Verification items for the finished model (mm, model axes). Face numbers are marked on the shaded views. A direction names the side the tool comes from. Coordinates: 2 decimals unless noted, no trailing zeros. Write each loop counter-clockwise with the first axis right and the second up, starting at its lowest first coordinate (ties: lowest second). Pieces come first, ordered by that corner, then holes. Notation, with made-up numbers: (37, 50.5) -> (56, 50.5) arc R33 cw to (56, 81.5) -> close; hole circle Ø10 at (15.5, 86.5). An arc over 180 degrees is marked (long way). Write item = value, one per line. Start each with the question number.
(1) Section check A-A (z = -26). Record the cut outline in (x, y), plus the area to 3 significant figures.
(2) Section check C-C (y = 25.5). Record the cut outline in (x, z).
(3) Gauge pin test, flat ends, axial feed: pin 1 Ø3 at (x, z) = (2.92, -26) entering from +Y; pin 2 Ø4 at (y, z) = (26.27, -13.5) entering from +X; pin 3 Ø5 at (x, z) = (5, -10.5) entering from +Y; pin 4 Ø7 at (x, y) = (4.5, 21) entering from -Z. Record the tip position at first contact, or that the pin passes through.
(4) Section check D-D (x = 2.92). Record the cut outline in (y, z), plus the area to 3 significant figures.
(5) Mould release check, pull along Z, two halves, no side actions. Record for the marked faces 4, 5 and 6: released by +Z, released by -Z, zero draft, split by the parting line, or undercut.
(6) Set-up check for the marked faces 1, 2 and 3: record each of +Z, -Z, +X, -X, +Y, -Y from which the full face is reachable in a straight line by a thin tool's end or side.
(7) Material ranges on probe 1 along Z at (x, y) = (6.75, 2); probe 2 along Y at (x, z) = (5, 5.5); probe 3 along Z at (x, y) = (1.25, 6.5), recorded low to high. Write a range as [from, to].
(8) Section check B-B (z = -17). Record the cut outline in (x, y), plus the area to 3 significant figures.
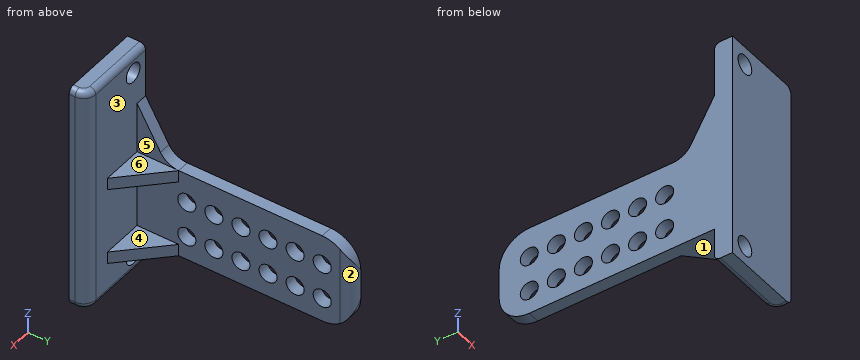
```python
from build123d import *

# Parameters (mm, degrees)
SKETCH_1_R          = 1.5
EXTRUDE_1_DEPTH     = 2
FILLET_1_R          = 2
SKETCH_2_W          = 13.65
SKETCH_2_H          = 38.14
EXTRUDE_2_DEPTH     = 3
SKETCH_5_R          = 1.6
CUT_EXTRUDE_1_DEPTH = 51.34658541
FILLET_5_R          = 2
FILLET_6_R          = 1
RIB_5_REACH         = 45.465
SKETCH_6_WALL_W     = 98.727749582
SKETCH_6_WALL_H     = 2
RIB_8_REACH         = 52.268
SKETCH_8_WALL_W     = 112.334064404
SKETCH_8_WALL_H     = 2


with BuildPart() as part:
    # 草图1 → 凸台-拉伸1 (new body)
    with BuildSketch(Plane(origin=(0, 0, 0), x_dir=(0, 0, -1), z_dir=(1, 0, 0))):
        with BuildLine():
            Line((8.5, 6.92820323), (8.5, 30.773589654))
            ThreePointArc((8.5, 30.773589654), (9.964466094, 34.30912356), (13.5, 35.773589654))
            Line((13.5, 35.773589654), (18.5, 35.773589654))
            ThreePointArc((18.5, 35.773589654), (22.035533906, 34.30912356), (23.5, 30.773589654))
            Line((23.5, 30.773589654), (23.5, 0))
            Line((23.5, 0), (0, 0))
            Line((0, 0), (6.75, 3.897114317))
            ThreePointArc((6.75, 3.897114317), (8.031088913, 5.17820323), (8.5, 6.92820323))
        make_face()
        with Locations((19.5, 30.773589654)):
            Circle(SKETCH_1_R, mode=Mode.SUBTRACT)
        with Locations((13.5, 30.773589654)):
            Circle(SKETCH_1_R, mode=Mode.SUBTRACT)
        with Locations((19.5, 26.273589654)):
            Circle(SKETCH_1_R, mode=Mode.SUBTRACT)
        with Locations((13.5, 26.273589654)):
            Circle(SKETCH_1_R, mode=Mode.SUBTRACT)
        with Locations((19.5, 21.773589654)):
            Circle(SKETCH_1_R, mode=Mode.SUBTRACT)
        with Locations((13.5, 21.773589654)):
            Circle(SKETCH_1_R, mode=Mode.SUBTRACT)
        with Locations((19.5, 17.273589654)):
            Circle(SKETCH_1_R, mode=Mode.SUBTRACT)
        with Locations((13.5, 17.273589654)):
            Circle(SKETCH_1_R, mode=Mode.SUBTRACT)
        with Locations((19.5, 12.773589654)):
            Circle(SKETCH_1_R, mode=Mode.SUBTRACT)
        with Locations((13.5, 12.773589654)):
            Circle(SKETCH_1_R, mode=Mode.SUBTRACT)
        with Locations((19.5, 8.273589654)):
            Circle(SKETCH_1_R, mode=Mode.SUBTRACT)
        with Locations((13.5, 8.273589654)):
            Circle(SKETCH_1_R, mode=Mode.SUBTRACT)
    extrude(amount=EXTRUDE_1_DEPTH)

    # 圆角1
    # the kernel refuses this fillet: 2 mm, written as the material it takes off along each edge
    with BuildSketch(Plane(origin=(2, 35.773589654, -8.5), x_dir=(-1, 0, 0), z_dir=(0, 0, -1))) as fillet_1_piece_1:
        with BuildLine():
            CenterArc((FILLET_1_R, -FILLET_1_R), FILLET_1_R, 90, 90)
            Line((0, -FILLET_1_R), (0, 0))
            Line((0, 0), (FILLET_1_R, 0))
        make_face()
    extrude(amount=15, mode=Mode.SUBTRACT)

    # 草图2 → 凸台-拉伸2 (add)
    with BuildSketch(Plane.XZ):
        with Locations((6.825, -10)):
            Rectangle(SKETCH_2_W, SKETCH_2_H)
    extrude(amount=EXTRUDE_2_DEPTH)

    # 草图5 → 切除-拉伸1 (cut, through all)
    with BuildSketch(Plane.XZ.offset(3)):
        with Locations(Location((2.92, 6, 0), (0, 0, 270))):
            Circle(SKETCH_5_R)
        with Locations(Location((2.92, -26, 0), (0, 0, 270))):
            Circle(SKETCH_5_R)
    extrude(amount=-CUT_EXTRUDE_1_DEPTH, mode=Mode.SUBTRACT)

    # 圆角5
    fillet_5_edges = [part.edges().sort_by_distance(p)[0] for p in [
        (13.65, 0, -10),
    ]]
    fillet(fillet_5_edges, radius=FILLET_5_R)

    # 圆角6
    fillet_6_edges = [part.edges().sort_by_distance(p)[0] for p in [
        (5.825, 0, 9.07),
        (13.064213562, -0.585786438, 9.07),
        (13.064213562, -0.585786438, -29.07),
        (5.825, 0, -29.07),
        (13.65, -2.5, -29.07),
        (13.65, -2.5, 9.07),
    ]]
    fillet(fillet_6_edges, radius=FILLET_6_R)

    # 草图6 wall → 筋5 (add, up to next)
    with BuildSketch(Plane(origin=(5.464101615, 3.464101615, -8.5), x_dir=(0.707106781187, -0.707106781187, 0), z_dir=(0.707106781187, 0.707106781187, 0)), mode=Mode.PRIVATE) as rib_5_sk1:
        with Locations((0, 1)):
            Rectangle(SKETCH_6_WALL_W, SKETCH_6_WALL_H)
    rib_5_tool1 = extrude(rib_5_sk1.sketch, amount=-RIB_5_REACH, mode=Mode.PRIVATE) - part.part
    add(rib_5_tool1.solids().sort_by_distance((5.464101615, 3.464101615, -8.5))[0])

    # 草图8 wall → 筋8 (add, up to next)
    with BuildSketch(Plane(origin=(5.464101615, 3.464101615, -23.5), x_dir=(0.707106781187, -0.707106781187, 0), z_dir=(-0.707106781187, -0.707106781187, 0)), mode=Mode.PRIVATE) as rib_8_sk1:
        with Locations((0, 1)):
            Rectangle(SKETCH_8_WALL_W, SKETCH_8_WALL_H)
    rib_8_tool1 = extrude(rib_8_sk1.sketch, amount=RIB_8_REACH, mode=Mode.PRIVATE) - part.part
    add(rib_8_tool1.solids().sort_by_distance((5.464101615, 3.464101615, -23.5))[0])


solid = part.part
```
Response:
q1.outline = (0, -3) -> (1.32, -3) -> (1.32, 0) -> (0, 0) -> close; (4.52, -3) -> (13.65, -3) -> (13.65, -2) arc R2 ccw to (11.65, 0) -> (4.52, 0) -> close
q1.area = 30.5 mm2
q2.outline = (0, -23.5) -> (2, -23.5) -> (2, -20.79) -> (0, -20.79) -> close; (0, -18.21) -> (2, -18.21) -> (2, -14.79) -> (0, -14.79) -> close; (0, -12.21) -> (2, -12.21) -> (2, -8.5) -> (0, -8.5) -> close
q3.pin_1 = through
q3.pin_2 = 2
q3.pin_3 = 6.43
q3.pin_4 = -23.5
q4.outline = (-3, -29.07) -> (-1, -29.07) arc R1 ccw to (0, -28.07) -> (0, -27.6) -> (-3, -27.6) -> close; (-3, -24.4) -> (0, -24.4) -> (0, -23.5) -> (6.01, -23.5) -> (6.01, -21.5) -> (0, -21.5) -> (0, -10.5) -> (6.01, -10.5) -> (6.01, -8.5) -> (0, -8.5) -> (0, 4.4) -> (-3, 4.4) -> close; (-3, 7.6) -> (0, 7.6) -> (0, 8.07) arc R1 ccw to (-1, 9.07) -> (-3, 9.07) -> close
q4.area = 119 mm2
q5.face_4 = undercut
q5.face_5 = zero draft
q5.face_6 = released by +Z
q6.face_1 = -Z, +X, -X, +Y
q6.face_2 = +Z, -Z, +X, +Y
q6.face_3 = +X, +Y
q7.probe_1 = [-23.5, -21.5], [-10.5, -8.5]
q7.probe_2 = [-3, 0]
q7.probe_3 = [-23.5, -8.47]
q8.outline = (0, -3) -> (13.65, -3) -> (13.65, -2) arc R2 ccw to (11.65, 0) -> (2, 0) -> (2, 33.77) arc R2 ccw to (0, 35.77) -> close
q8.area = 111 mm2
